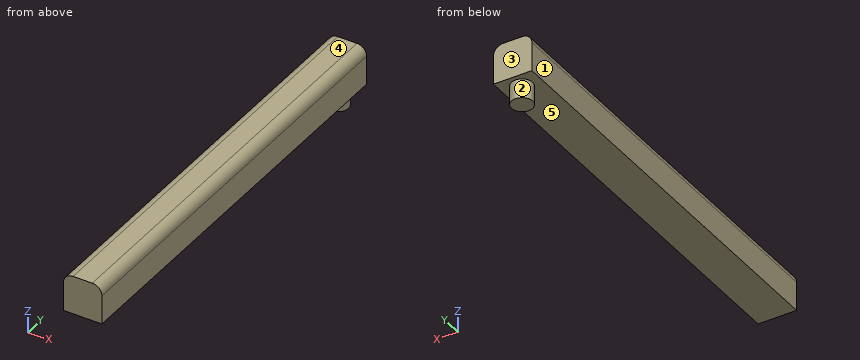
from build123d import *

# Parameters (mm, degrees)
SKETCH2_W           = 10
SKETCH2_H           = 110
BOSS_EXTRUDE1_DEPTH = 10
SKETCH3_R           = 2.75
BOSS_EXTRUDE2_DEPTH = 5
FILLET2_R           = 2.5


with BuildPart() as part:
    # Sketch2 → Boss-Extrude1 (new body)
    with BuildSketch(Plane.XY):
        with Locations((5, 55)):
            Rectangle(SKETCH2_W, SKETCH2_H)
    extrude(amount=BOSS_EXTRUDE1_DEPTH)

    # Sketch3 → Boss-Extrude2 (add)
    with BuildSketch(Plane(origin=(0, 0, 0), x_dir=(-1, 0, 0), z_dir=(0, 0, -1))):
        with Locations((-5, 106.074407224)):
            Circle(SKETCH3_R)
    extrude(amount=BOSS_EXTRUDE2_DEPTH)

    # Fillet2
    fillet2_edges = [part.edges().sort_by_distance(p)[0] for p in [
        (0, 55, 10),
        (10, 55, 10),
    ]]
    fillet(fillet2_edges, radius=FILLET2_R)


solid = part.part
Could you check a few things on this model? Use its own coordinates, in mm. Face numbers are marked on the shaded views. A direction names the side the tool comes from. Coordinates: 2 decimals unless noted, no trailing zeros. Order: outer loops, then holes, each group sorted by start corner. A loop starts at its lowest first (then second) coordinate and runs counter-clockwise, first axis right, second up.
Q1. Thinking about a two-plate mould opening in Z: for the marked faces 3, 4 and 5, which applies, released by +Z, released by -Z, zero draft, split by the parting line, or undercut?
Q2. Suppose I cut it at A-A on y = 14.5. Please give me the cut outline in (x, z), and give its area (3 significant figures).
Q3. Suppose I cut it at B-B on x = 5. Please give me the cut outline in (y, z), and give its area (3 significant figures).
Q4. Please list where these lines run through material, in increasing order: L1, parallel to Z at x = 4, y = 56.5; L2, parallel to X at y = 104, z = -3.5; L3, parallel to Y at x = 7.5, z = -1.
Q5. Which directions (+Z, -Z, +X, -X, +Y, -Y) give clear straight access to the entire face, cutting with the end or side of a thin tool? Please do the marked faces 1 and 2.
Q6. Will this pin go through, and if not, where does the flat tip stop? pin 1 (1 mm diameter, centred on x = 2.5, z = -1.5, fed in from +Y).
Answer:
1. face 3: zero draft
1. face 4: released by +Z
1. face 5: released by -Z
2. outline: (0, 0) - (10, 0) - (10, 7.5) arc R2.5 ccw to (7.5, 10) - (2.5, 10) arc R2.5 ccw to (0, 7.5) - close
2. area: 97.3 mm2
3. outline: (0, 0) - (103.32, 0) - (103.32, -5) - (108.82, -5) - (108.82, 0) - (110, 0) - (110, 10) - (0, 10) - close
3. area: 1,130 mm2
4. L1: z = 0 to 10
4. L2: x = 3.19 to 6.81
4. L3: y = 104.93 to 107.22
5. face 1: +Z, -Z, -X, +Y, -Y
5. face 2: -Z
6. pin 1: stops at y = 107.96
